Input: part model. Units: mm. Frame: model coordinates. Face numbers are marked on the shaded views. A direction names the side the tool comes from. Round coordinates to 2 decimals unless told otherwise and drop trailing zeros. Loops run counter-clockwise (first coordinate to the right, second up) from the corner with the lowest first, then second, coordinate; pieces in that order, holes last.
(1) Cut plane C-C, the plane y = 43.5. Output: boundary loops of the cut face in (x, z), and give its area (3 significant figures).
(2) Cut plane B-B, the plane x = 64.5. Output: boundary loops of the cut face in (y, z), and give its area (3 significant figures).
(3) Draft query along X for the marked faces 1, 2, 3 and 4. Return one class per face: released by +X, released by -X, zero draft, split by the parting line, or undercut.
(4) Line query: line 1 (X direction, y = 32, z = -4); line 2 (Z direction, x = 55.5, y = 68); line 3 (Z direction, x = 64.5, y = 9.5). Output: solid intervals per line, ascending.
(5) Access query for the marked faces 5, 6 and 7. Directions: +Z, -Z, +X, -X, +Y, -Y. A direction counts if a zero-diameter tool reaches every point of the face in a straight line with its end or side. Return the directions, or none.
(6) Cut plane D-D, the plane x = 45.5. Output: boundary loops of the cut face in (y, z).
(7) First-contact query: pin 1 Ø6 at (x, z) = (36.5, -40.5) entering from -Y; pin 2 Ø8 at (x, y) = (60, 13) entering from +Z; pin 3 Ø18 at (y, z) = (23.5, 1.5) entering from -X; pin 4 Ø10 at (y, z) = (20, -12.5) entering from +X. Flat tips, straight axial feed; report the tip coordinate or a pass-through.
(8) Cut plane A-A, the plane z = -5.5. Output: boundary loops of the cut face in (x, y).
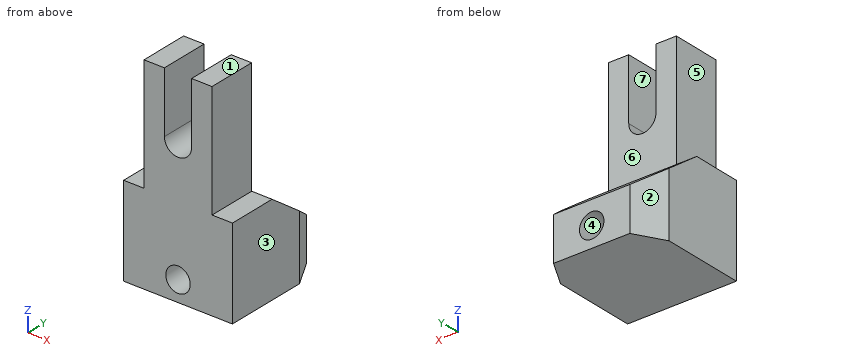
from build123d import *

# Parameters (mm, degrees)
CROQUIS1_W              = 80
CROQUIS1_H              = 150
SALIENTE_EXTRUIR1_DEPTH = 82
CORTAR_EXTRUIR1_DEPTH   = 150
CROQUIS3_R              = 9
CROQUIS3_W              = 12
CROQUIS3_H              = 84
CROQUIS3_W_2            = 3
CORTAR_EXTRUIR2_DEPTH   = 150
CORTAR_EXTRUIR3_DEPTH   = 80


with BuildPart() as part:
    # Croquis1 → Saliente-Extruir1 (new body)
    with BuildSketch(Plane(origin=(0, 0, 0), x_dir=(1, 0, 0), z_dir=(0, 1, 0))):
        with Locations((58.762376238, 47.339108911)):
            Rectangle(CROQUIS1_W, CROQUIS1_H)
    extrude(amount=SALIENTE_EXTRUIR1_DEPTH)

    # Croquis2 → Cortar-Extruir1 (cut)
    with BuildSketch(Plane(origin=(0, 0, -122.339108911), x_dir=(-1, 0, 0), z_dir=(0, 0, -1))):
        Polygon((-98.762376238, 82), (-98.762376238, 61), (-86.762376238, 82), align=None)
        Polygon((-18.762376238, 82), (-30.762376238, 82), (-18.762376238, 61), align=None)
    extrude(amount=-CORTAR_EXTRUIR1_DEPTH, mode=Mode.SUBTRACT)

    # Croquis3 → Cortar-Extruir2 (cut)
    with BuildSketch(Plane(origin=(0, 82, 0), x_dir=(1, 0, 0), z_dir=(0, 1, 0))):
        with Locations((58.762376238, 107.339108911)):
            Circle(CROQUIS3_R)
        with BuildLine():
            ThreePointArc((68.762376238, 17.339108911), (58.762376238, 27.339108911), (48.762376238, 17.339108911))
            Line((48.762376238, 17.339108911), (48.762376238, -27.660891089))
            Line((48.762376238, -27.660891089), (68.762376238, -27.660891089))
            Line((68.762376238, -27.660891089), (68.762376238, 17.339108911))
        make_face()
        with Locations((24.762376238, 14.339108911)):
            Rectangle(CROQUIS3_W, CROQUIS3_H)
        with Locations((32.262376238, 14.339108911)):
            Rectangle(CROQUIS3_W_2, CROQUIS3_H)
        with Locations((92.762376238, 14.339108911)):
            Rectangle(CROQUIS3_W, CROQUIS3_H)
        with Locations((85.262376238, 14.339108911)):
            Rectangle(CROQUIS3_W_2, CROQUIS3_H)
    extrude(amount=-CORTAR_EXTRUIR2_DEPTH, mode=Mode.SUBTRACT)

    # Croquis4 → Cortar-Extruir3 (cut)
    with BuildSketch(Plane(origin=(98.762376238, 0, 0), x_dir=(0, 0, -1), z_dir=(1, 0, 0))):
        Polygon((-27.660891089, 36), (56.339108911, 36), (90.339108911, 82), (-27.660891089, 82), align=None)
    extrude(amount=-CORTAR_EXTRUIR3_DEPTH, mode=Mode.SUBTRACT)


solid = part.part
Reported:
1. outline: (18.76, -122.34) - (98.76, -122.34) - (98.76, -61.88) - (18.76, -61.88) - close; hole circle Ø18 at (58.76, -107.34)
1. area: 4,580 mm2
2. outline: (0, -122.34) - (82, -122.34) - (82, -114.27) - (0, -114.27) - close; (0, -100.41) - (82, -100.41) - (82, -90.34) - (36, -56.34) - (36, -25.53) - (0, -25.53) - close
2. area: 4,600 mm2
3. face 1: zero draft
3. face 2: released by -X
3. face 3: released by +X
3. face 4: undercut
4. line 1: x = 33.76 to 48.76, 68.76 to 83.76
4. line 2: z = -122.34 to -115.73, -98.95 to -79.99
4. line 3: z = -122.34 to -114.27, -100.41 to -25.53
5. face 5: +Z, -X, +Y, -Y
5. face 6: +Z, +X, -X, +Y
5. face 7: +Z, +Y, -Y
6. outline: (0, -122.34) - (82, -122.34) - (82, -90.34) - (36, -56.34) - (36, 27.66) - (0, 27.66) - close
7. pin 1: stops at y = 0
7. pin 2: stops at z = -25.86
7. pin 3: stops at x = 33.76
7. pin 4: stops at x = 83.76
8. outline: (33.76, 0) - (48.76, 0) - (48.76, 36) - (33.76, 36) - close; (68.76, 0) - (83.76, 0) - (83.76, 36) - (68.76, 36) - close
